Drawing for the job (mm, zero at the part's lowest x, y, z). Coordinates: 2 decimals unless noted, no trailing zeros. Write each loop counter-clockwise with the first axis right and the second up, starting at its lowest first coordinate (ties: lowest second). Pieces come first, ordered by that corner, then holes. Notation, with made-up numbers: (71.25, 17.5) -> (77.25, 17.5) arc R19 cw to (77.25, 46.5) -> close; hole circle Ø7 at (55.25, 68). An arc over 180 degrees is marked (long way). Write item = value, one per line. Start each with the question number.
Q1. Pin check, flat tips, straight feed: P1, Ø3, axis at y = 34, z = 1.5, coming from the +X side; P2, Ø3, axis at y = 211, z = 1, coming from the -X side; P3, Ø3, axis at x = 98, y = 125, coming from the -Z side. Stop position of each tip, or through.
Q2. Band-saw the part on C-C, the plane y = 226. List the corners of the cut face in (x, z), plus the area to 3 significant figures.
Q3. Band-saw the part on B-B, the plane x = 166. List the corners of the cut face in (y, z), plus the area to 3 significant figures.
Q4. Band-saw the part on A-A, the plane z = 3.75. List the corners of the cut face in (x, y), plus the area to 3 significant figures.
Q5. Probe line 1 (Y direction, x = 125, z = 2.15); line 2 (Y direction, x = 113, z = 0.95); line 3 (Y direction, x = 152, z = 3.3). List the from-to ranges inside material, lowest first.
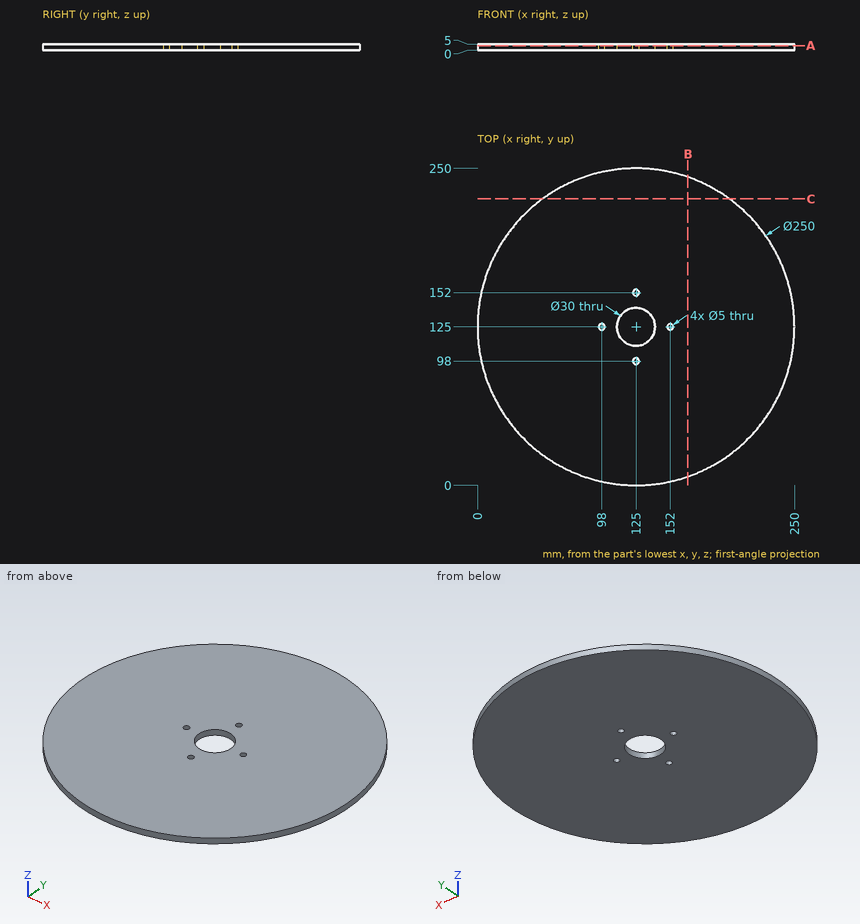
Ans:
q1.P1 = 212.26
q1.P2 = 32.89
q1.P3 = through
q2.outline = (51.35, 0) -> (198.65, 0) -> (198.65, 5) -> (51.35, 5) -> close
q2.area = 736 mm2
q3.outline = (6.92, 0) -> (243.08, 0) -> (243.08, 5) -> (6.92, 5) -> close
q3.area = 1,180 mm2
q4.outline = circle Ø250 at (125, 125); hole circle Ø5 at (98, 125); hole circle Ø30 at (125, 125); hole circle Ø5 at (125, 98); hole circle Ø5 at (125, 152); hole circle Ø5 at (152, 125)
q4.area = 48,300 mm2
q5.line_1 = 0 to 95.5, 100.5 to 110, 140 to 149.5, 154.5 to 250
q5.line_2 = 0.58 to 116, 134 to 249.42
q5.line_3 = 2.95 to 122.5, 127.5 to 247.05
